from build123d import *

# Parameters (mm, degrees)
SKETCH_1_R          = 1.5
EXTRUDE_1_DEPTH     = 20
SKETCH_2_R          = 2.5
CUT_EXTRUDE_1_DEPTH = 20


with BuildPart() as part:
    # Sketch 1 → Extrude 1 (new body)
    with BuildSketch(Plane.XY):
        with BuildLine():
            Line((-4.826530612, 15.115646259), (-10.326530612, 15.115646259))
            Line((-10.326530612, 15.115646259), (-10.326530612, -9.884353741))
            Line((-10.326530612, -9.884353741), (-20.326530612, -9.884353741))
            Line((-20.326530612, -9.884353741), (-20.326530612, -17.884353741))
            Line((-20.326530612, -17.884353741), (21.673469388, -17.884353741))
            Line((21.673469388, -17.884353741), (21.673469388, -9.884353741))
            Line((21.673469388, -9.884353741), (11.673469388, -9.884353741))
            Line((11.673469388, -9.884353741), (11.673469388, 15.115646259))
            Line((11.673469388, 15.115646259), (6.205006293, 15.115646259))
            Line((6.205006293, 15.115646259), (6.205006293, 4.115646259))
            Line((6.205006293, 4.115646259), (6.173469388, 4.115646259))
            ThreePointArc((6.173469388, 4.115646259), (0.673469388, -1.384353741), (-4.826530612, 4.115646259))
            Line((-4.826530612, 4.115646259), (-4.826530612, 15.115646259))
        make_face()
        with Locations((0.673469388, -3.884353741)):
            Circle(SKETCH_1_R, mode=Mode.SUBTRACT)
        with Locations((-7.326530612, 4.115646259)):
            Circle(SKETCH_1_R, mode=Mode.SUBTRACT)
        with Locations((8.673469388, 4.115646259)):
            Circle(SKETCH_1_R, mode=Mode.SUBTRACT)
    extrude(amount=EXTRUDE_1_DEPTH)

    # Sketch 2 → Cut-Extrude 1 (cut)
    with BuildSketch(Plane(origin=(0, -9.884353741, 0), x_dir=(1, 0, 0), z_dir=(0, 1, 0))):
        with Locations(Location((16.673469388, -10, 0), (0, 0, 270))):
            Circle(SKETCH_2_R)
        with Locations(Location((-15.326530612, -10, 0), (0, 0, 270))):
            Circle(SKETCH_2_R)
    extrude(amount=-CUT_EXTRUDE_1_DEPTH, mode=Mode.SUBTRACT)


solid = part.part
For this review, take the finished solid that the model builds, in its own axes (mm). A direction names the side the tool comes from. Give positions to 0.01 mm unless a question says otherwise; leave off trailing zeros. Order: outer loops, then holes, each group sorted by start corner. A loop starts at its lowest first (then second) coordinate and runs counter-clockwise, first axis right, second up. Notation, with made-up numbers: (31, -18.5) - (42, -18.5) arc R23 ccw to (42, -7.5) - close; hole circle Ø5 at (42, 57). An arc over 180 degrees is marked (long way). Answer as a JSON object with one key per item and string values. Group by question number.
Item 1: Take a section at B-B on z = 9.5. Give the boundary of the cut face in (x, y) (3 decimals).
Item 2: Wall thickness on line 1 along X through (y, z) = (7, 11.5) (3 decimals); line 2 along X through (y, z) = (3, 13.5); line 3 along Y through (x, z) = (13, 18.75): over which ranges is each line inside the solid? List them lowest first.
Item 3: Machinability: for faces 4 (the flat face through (17.9, -9.884, 7.6)), 5 (the flat face through (-4.827, 10, 10)), 6 (the flat face through (-14.1, -9.884, 7.6)), which of the approach directions +Z, -Z, +X, -X, +Y, -Y give a long, thin tool a straight path to every point of the face, cutting with its end or side? Answer none if there is none.
Item 4: Take a section at D-D on z = 13.75. Give the boundary of the cut face in (x, y) (3 decimals), and give its area (3 significant figures).
Item 5: Clearance check with flat-ended pins moving along their axes: pin 1 Ø3 at (x, z) = (17, 7) entering from +Y; pin 2 Ø1.8 at (x, y) = (-7.33, 4.12) entering from -Z; pin 3 Ø5 at (y, z) = (3.5, 14.5) entering from +X; pin 4 Ø10 at (y, z) = (4.5, 6.5) entering from -X. State where each tip first meets the part, or that it passes through.
Item 6: Draft analysis for pull direction Y (two halves, no side actions). For faces 1 (the cylindrical face through (-8.517, 3.203, 9.86)), 2 (the cylindrical face through (14.233, -13.828, 9.458)), 3 (the flat face through (0, -17.884, 10)), state which applies: pulls with the +Y half, pulls with the -Y half, needs draft (parallel to the pull), parting line crosses it, or undercut.
Item 7: Take a section at C-C on x = -17. Give the boundary of the cut face in (y, z), and give its area (3 significant figures).
Item 8: Take a section at A-A on y = 13.5. Give the boundary of the cut face in (x, z) (3 decimals).
Reported:
{
 "1": {"outline": "(-20.327, -17.884) - (-17.776, -17.884) - (-17.776, -9.884) - (-20.327, -9.884) - close; (-12.877, -17.884) - (14.224, -17.884) - (14.224, -9.884) - (11.673, -9.884) - (11.673, 15.116) - (6.205, 15.116) - (6.205, 4.116) - (6.173, 4.116) arc R5.5 cw to (-4.827, 4.116) - (-4.827, 15.116) - (-10.327, 15.116) - (-10.327, -9.884) - (-12.877, -9.884) - close; (19.123, -17.884) - (21.673, -17.884) - (21.673, -9.884) - (19.123, -9.884) - close; hole circle Ø3 at (-7.327, 4.116); hole circle Ø3 at (0.673, -3.884); hole circle Ø3 at (8.673, 4.116)"},
 "2": {"line 1": "-10.327 to -4.827, 6.205 to 11.673", "line 2": "-10.33 to -8.33, -6.32 to -4.71, 6.06 to 7.67, 9.68 to 11.67", "line 3": "-17.88 to -9.88"},
 "3": {"face 4": "+Z, -Z, +X, +Y", "face 5": "+Z, -Z, +Y", "face 6": "+Z, -Z, -X, +Y"},
 "4": {"outline": "(-20.327, -17.884) - (21.673, -17.884) - (21.673, -9.884) - (11.673, -9.884) - (11.673, 15.116) - (6.205, 15.116) - (6.205, 4.116) - (6.173, 4.116) arc R5.5 cw to (-4.827, 4.116) - (-4.827, 15.116) - (-10.327, 15.116) - (-10.327, -9.884) - (-20.327, -9.884) - close; hole circle Ø3 at (-7.327, 4.116); hole circle Ø3 at (0.673, -3.884); hole circle Ø3 at (8.673, 4.116)", "area": "696 mm^2"},
 "5": {"pin 1": "y = -9.88", "pin 2": "through", "pin 3": "x = 11.67", "pin 4": "x = -10.33"},
 "6": {"face 1": "undercut", "face 2": "needs draft", "face 3": "pulls with the -Y half"},
 "7": {"outline": "(-17.88, 0) - (-9.88, 0) - (-9.88, 8.14) - (-17.88, 8.14) - close; (-17.88, 11.86) - (-9.88, 11.86) - (-9.88, 20) - (-17.88, 20) - close", "area": "130 mm^2"},
 "8": {"outline": "(-10.327, 0) - (-4.827, 0) - (-4.827, 20) - (-10.327, 20) - close; (6.205, 0) - (11.673, 0) - (11.673, 20) - (6.205, 20) - close"}
}
